```python
from build123d import *

# Parameters (mm, degrees)
SKETCH1_W           = 572
SKETCH1_H           = 197
BOSS_EXTRUDE1_DEPTH = 25
BOSS_EXTRUDE1_TAPER = 1
SKETCH2_W           = 532
SKETCH2_H           = 157
CUT_EXTRUDE1_DEPTH  = 3
CUT_EXTRUDE1_TAPER  = 1
SKETCH4_W           = 532
SKETCH4_H           = 156.89526961
SKETCH4_W_2         = 515
SKETCH4_H_2         = 140
CUT_EXTRUDE2_DEPTH  = 7
CUT_EXTRUDE2_TAPER  = 1


with BuildPart() as part:
    # Sketch1 → Boss-Extrude1 (new body)
    with BuildSketch(Plane(origin=(0, 0, 0), x_dir=(1, 0, 0), z_dir=(0, 1, 0))):
        Rectangle(SKETCH1_W, SKETCH1_H)
    extrude(amount=BOSS_EXTRUDE1_DEPTH, taper=BOSS_EXTRUDE1_TAPER)

    # Sketch2 → Cut-Extrude1 (cut)
    with BuildSketch(Plane(origin=(0, 25, 0), x_dir=(1, 0, 0), z_dir=(0, 1, 0))):
        Rectangle(SKETCH2_W, SKETCH2_H)
    extrude(amount=-CUT_EXTRUDE1_DEPTH, taper=CUT_EXTRUDE1_TAPER, mode=Mode.SUBTRACT)

    # Sketch4 → Cut-Extrude2 (cut)
    with BuildSketch(Plane(origin=(0, 22, 0), x_dir=(1, 0, 0), z_dir=(0, 1, 0))):
        Rectangle(SKETCH4_W, SKETCH4_H)
        Rectangle(SKETCH4_W_2, SKETCH4_H_2, mode=Mode.SUBTRACT)
    extrude(amount=-CUT_EXTRUDE2_DEPTH, taper=CUT_EXTRUDE2_TAPER, mode=Mode.SUBTRACT)


solid = part.part
```
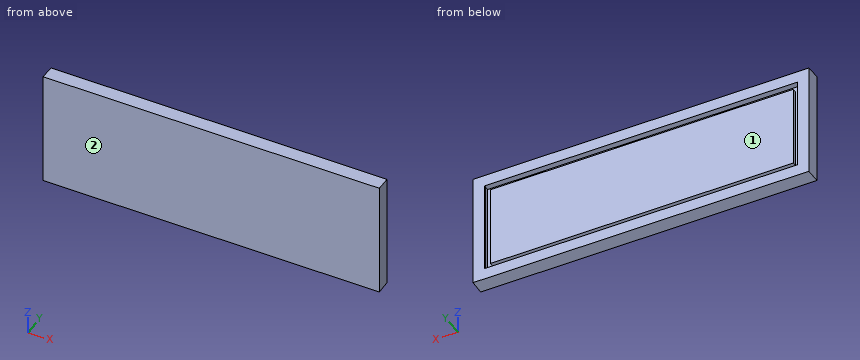
Input: part model. Units: mm. Frame: model coordinates. Face numbers are marked on the shaded views. Round coordinates to 2 decimals unless told otherwise and drop trailing zeros. One line per item, written item: value. Start each with the question number.
(1) Draft query along X for the marked faces 1 and 2. Return one class per face: +X half, -X half, draft (parallel to the pull), parting line (faces both ways), or undercut.
(2) Contact query for flat-ended pins moving along their axis: P1, Ø12, axis at x = 107.5, y = 13.5, coming from the -Z side; P2, Ø4, axis at x = -19, z = -46.5, coming from the +Y side; P3, Ø2, axis at x = -179, y = 3.5, coming from the +Z side. Output: stop coordinate, or through.
(3) Ray query, line 1 (X direction, y = 19.5, z = 66); line 2 (Z direction, x = -25, y = 21); line 3 (Z direction, x = -110, y = 18.5). Return the intervals inside material, ascending. Write a range as [from, to].
Results below:
1. face 1: undercut
1. face 2: draft
2. P1: z = -98.37
2. P2: y = 22
2. P3: z = 98.46
3. line 1: [-285.66, -265.96], [-257.54, 257.54], [265.96, 285.66]
3. line 2: [-98.13, -78.43], [-70.02, 70.02], [78.43, 98.13]
3. line 3: [-98.18, -78.39], [-70.06, 70.06], [78.39, 98.18]
